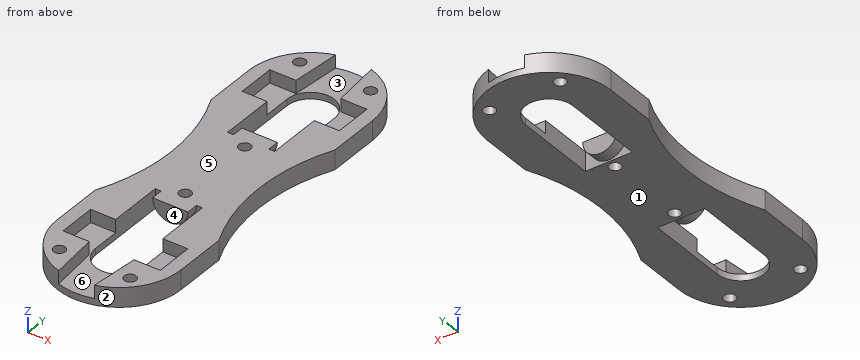
```python
from build123d import *

# Parameters (mm, degrees)
SKETCH_1_R          = 1
EXTRUDE_1_DEPTH     = 3.3
CUT_EXTRUDE_1_DEPTH = 2.2
EXTRUDE_2_DEPTH     = 2


with BuildPart() as part:
    # 草图1 → 凸台-拉伸1 (new body)
    with BuildSketch(Plane.XY):
        with BuildLine():
            Line((10.5, -13.638181697), (10.5, -22.5))
            ThreePointArc((10.5, -22.5), (0, -33), (-10.5, -22.5))
            Line((-10.5, -22.5), (-10.5, -13.638181697))
            ThreePointArc((-10.5, -13.638181697), (-7.5, 0), (-10.5, 13.638181697))
            Line((-10.5, 13.638181697), (-10.5, 22.5))
            ThreePointArc((-10.5, 22.5), (0, 33), (10.5, 22.5))
            Line((10.5, 22.5), (10.5, 13.638181697))
            ThreePointArc((10.5, 13.638181697), (7.5, 0), (10.5, -13.638181697))
        make_face()
        with Locations((0, 7)):
            Circle(SKETCH_1_R, mode=Mode.SUBTRACT)
        with Locations((0, -7)):
            Circle(SKETCH_1_R, mode=Mode.SUBTRACT)
        with Locations((-6, 28.25)):
            Circle(SKETCH_1_R, mode=Mode.SUBTRACT)
        with Locations((6, 28.25)):
            Circle(SKETCH_1_R, mode=Mode.SUBTRACT)
        with Locations((6, -28.25)):
            Circle(SKETCH_1_R, mode=Mode.SUBTRACT)
        with Locations((-6, -28.25)):
            Circle(SKETCH_1_R, mode=Mode.SUBTRACT)
        with BuildLine():
            Line((-4, -22.499999544), (-4, -8.5))
            Line((-4, -8.5), (4, -8.5))
            Line((4, -8.5), (4, -22.500000456))
            ThreePointArc((4, -22.500000456), (-4.56e-07, -26.5), (-4, -22.499999544))
        make_face(mode=Mode.SUBTRACT)
        with BuildLine():
            Line((-4, 22.499999544), (-4, 8.5))
            Line((-4, 8.5), (4, 8.5))
            Line((4, 8.5), (4, 22.500000456))
            ThreePointArc((4, 22.500000456), (-4.56e-07, 26.5), (-4, 22.499999544))
        make_face(mode=Mode.SUBTRACT)
    extrude(amount=EXTRUDE_1_DEPTH)

    # 草图2 → 切除-拉伸1 (cut)
    with BuildSketch(Plane.XY.offset(3.3)):
        Polygon((-3.8, 24.3), (-2.871447866, 34.3), (2.871447866, 34.3), (3.8, 24.3), (8.25, 24.3), (8.25, 17.8), (-8.25, 17.8), (-8.25, 24.3), align=None)
        Polygon((3.8, -24.3), (8.25, -24.3), (8.25, -17.8), (-8.25, -17.8), (-8.25, -24.3), (-3.8, -24.3), (-2.871447866, -34.3), (2.871447866, -34.3), align=None)
    extrude(amount=-CUT_EXTRUDE_1_DEPTH, mode=Mode.SUBTRACT)

    # 草图3 → 凸台-拉伸2 (add)
    with BuildSketch(Plane(origin=(0, 8.5, 0), x_dir=(1, 0, 0), z_dir=(0, 1, 0))):
        with BuildLine():
            Line((-3, -3.3), (3, -3.3))
            ThreePointArc((3, -3.3), (0, -0.3), (-3, -3.3))
        make_face()
    extrude_2 = extrude(amount=EXTRUDE_2_DEPTH)

    # 镜向1: 凸台-拉伸2 across plane
    add(extrude_2.mirror(Plane.ZX))


solid = part.part
```
The model under review builds one solid part; all positions refer to its coordinate system, in mm. Face numbers are marked on the shaded views. A direction names the side the tool comes from. Round coordinates to 2 decimals unless told otherwise and drop trailing zeros. Write each loop counter-clockwise with the first axis right and the second up, starting at its lowest first coordinate (ties: lowest second). Pieces come first, ordered by that corner, then holes. Notation, with made-up numbers: (-17, 1.25) - (4, 1.25) arc R32 ccw to (4, 35.25) - close; hole circle Ø11 at (2, -32). An arc over 180 degrees is marked (long way). Answer as CSV lines item,"result". Start each with the question number.
(1) We need section D-D on x = -6. State the section outline as (y, z) points, plus the area to 3 significant figures.
(2) For pin 1 Ø1.1 at (x, z) = (5.5, 2.5) entering from +Y; pin 2 Ø3 at (x, y) = (3.5, 19) entering from +Z; pin 3 Ø1 at (x, z) = (7, 2.5) entering from -Y; pin 4 Ø1 at (y, z) = (-12, 2) entering from -X, all flat-tipped, find the tip position at first contact; note any pin that passes through.
(3) We need section B-B on y = -16. State the section outline as (x, z) points, plus the area to 3 significant figures.
(4) To check wall thickness, follow line 1 (Y direction, x = 6, z = 2.1); line 2 (X direction, y = -14, z = 2.3); line 3 (Y direction, x = 6, z = 0.85). State the ranges of each line that lie inside material, in increasing order.
(5) Draft analysis for pull direction X (two halves, no side actions). For the marked faces 1, 2 and 3, state which applies: pulls with the +X half, pulls with the -X half, needs draft (parallel to the pull), parting line crosses it, or undercut.
(6) For the marked faces 4, 5 and 6, list the 3-axis set-ups (+Z, -Z, +X, -X, +Y, -Y) from which the entire face can be reached by the end or side of a thin tool; tool diameter is ignored.
(7) We need section C-C on y = -28.25. State the section outline as (x, z) points, plus the area to 3 significant figures.
(8) We need section A-A on x = 0. State the section outline as (y, z) points.
Worked answers:
1,outline,"(-31.12, 0) - (-29.25, 0) - (-29.25, 3.3) - (-31.12, 3.3) - close; (-27.25, 0) - (27.25, 0) - (27.25, 3.3) - (24.3, 3.3) - (24.3, 1.1) - (17.8, 1.1) - (17.8, 3.3) - (-17.8, 3.3) - (-17.8, 1.1) - (-24.3, 1.1) - (-24.3, 3.3) - (-27.25, 3.3) - close; (29.25, 0) - (31.12, 0) - (31.12, 3.3) - (29.25, 3.3) - close"
1,area,"164 mm²"
2,pin 1,"y = 31.76"
2,pin 2,"z = 3.3"
2,pin 3,"y = -30.75"
2,pin 4,"x = -10"
3,outline,"(-10.5, 0) - (-4, 0) - (-4, 3.3) - (-10.5, 3.3) - close; (4, 0) - (10.5, 0) - (10.5, 3.3) - (4, 3.3) - close"
3,area,"42.9 mm²"
4,line 1,"-31.12 to -29.25, -27.25 to -24.3, -17.8 to 17.8, 24.3 to 27.25, 29.25 to 31.12"
4,line 2,"-10.5 to -4, 4 to 10.5"
4,line 3,"-31.12 to -29.25, -27.25 to 27.25, 29.25 to 31.12"
5,face 1,"needs draft"
5,face 2,"parting line crosses it"
5,face 3,"undercut"
6,face 4,"+Z, -Z"
6,face 5,"+Z, +X, -X, +Y, -Y"
6,face 6,"+Z"
7,outline,"(-8.79, 0) - (-7, 0) - (-7, 3.3) - (-8.79, 3.3) - close; (-5, 0) - (5, 0) - (5, 3.3) - (3.43, 3.3) - (3.43, 1.1) - (-3.43, 1.1) - (-3.43, 3.3) - (-5, 3.3) - close; (7, 0) - (8.79, 0) - (8.79, 3.3) - (7, 3.3) - close"
7,area,"29.7 mm²"
8,outline,"(-33, 0) - (-26.5, 0) - (-26.5, 1.1) - (-33, 1.1) - close; (-10.5, 0.3) - (-8.5, 0.3) - (-8.5, 0) - (-8, 0) - (-8, 3.3) - (-10.5, 3.3) - close; (-6, 0) - (6, 0) - (6, 3.3) - (-6, 3.3) - close; (8, 0) - (8.5, 0) - (8.5, 0.3) - (10.5, 0.3) - (10.5, 3.3) - (8, 3.3) - close; (26.5, 0) - (33, 0) - (33, 1.1) - (26.5, 1.1) - close"
